Check sheet for the modelled part. Datum: model origin and axes. Units: mm. A direction names the side the tool comes from. Give positions to 0.01 mm unless a question says otherwise; leave off trailing zeros. Write each loop counter-clockwise with the first axis right and the second up, starting at its lowest first coordinate (ties: lowest second). Pieces come first, ordered by that corner, then holes. Notation, with made-up numbers: M -23.5,-6 L -1.5,-6 A21 ccw -1.5,5 Z; hole C 37.5,56 d8. An arc over 180 degrees is marked long. One line per item, written item: value. Start each with the question number.
from build123d import *

# Parameters (mm, degrees)
SKETCH1_R           = 11
BOSS_EXTRUDE1_DEPTH = 36.1
SKETCH3_R           = 2.15
CUT_EXTRUDE1_DEPTH  = 17


with BuildPart() as part:
    # Sketch1 → Boss-Extrude1 (new body)
    with BuildSketch(Plane.XY):
        Polygon((-15, 15), (15, 15), (25, 15), (25, 5), (25, -15), (-25, -15), (-25, 5), (-25, 15), align=None)
        Circle(SKETCH1_R, mode=Mode.SUBTRACT)
    extrude(amount=BOSS_EXTRUDE1_DEPTH)

    # Sketch3 → Cut-Extrude1 (cut)
    with BuildSketch(Plane.XZ.offset(15)):
        with Locations((-17.5, 30.05)):
            Circle(SKETCH3_R)
        with Locations((17.5, 30.05)):
            Circle(SKETCH3_R)
        with Locations((17.5, 6.05)):
            Circle(SKETCH3_R)
        with Locations((-17.5, 6.05)):
            Circle(SKETCH3_R)
    extrude(amount=-CUT_EXTRUDE1_DEPTH, mode=Mode.SUBTRACT)


solid = part.part
1) Gauge pin test, flat end, axial feed: pin 1 (1.3 mm diameter, centred on x = -18.5, z = 30.5, fed in from -Y). Record the tip position at first contact, or that the pin passes through.
2) Cross-section at D-D (y = 5.5). Record the boundary of the cut face in (x, z), plus the area to 3 significant figures.
3) Cross-section at A-A (x = 0). Record the boundary of the cut face in (y, z).
4) Draft check along Y on faces 1 (the flat face through (17, 2, 6)), 2 (the cylindrical face through (-2.38, -10.74, 17.8)), 3 (the flat face through (25, 0, 18)). Enter one of: released by +Y, released by -Y, zero draft, split by the parting line, or undercut.
5) Cross-section at C-C (z = 6.05). Record the boundary of the cut face in (x, y), plus the area to 3 significant figures.
6) Tool access check on faces 4 (the cylindrical face through (17.22, -6.62, 32.18)), 5 (the flat face through (11.5, 0.2, 36.1)). Record the directions out of +Z, -Z, +X, -X, +Y, -Y that give a thin tool (end or side, any length) a straight path to the whole face; none if there is none.
7) Material ranges on L1, parallel to Z at x = -17.5, y = -9.25; L2, parallel to Y at x = 0, z = 20.5; L3, parallel to Z at x = -18, y = -12, recorded low to high. Write a range as from..to.
8) Cross-section at B-B (y = -10). Record the boundary of the cut face in (x, z), plus the area to 3 significant figures.
Data:
1. pin 1: stops at y = 2
2. outline: M -25,0 L -9.53,0 L -9.53,36.1 L -25,36.1 Z; M 9.53,0 L 25,0 L 25,36.1 L 9.53,36.1 Z
2. area: 1,120 mm2
3. outline: M -15,0 L -11,0 L -11,36.1 L -15,36.1 Z; M 11,0 L 15,0 L 15,36.1 L 11,36.1 Z
4. face 1: released by -Y
4. face 2: undercut
4. face 3: zero draft
5. outline: M -25,-15 L -19.65,-15 L -19.65,2 L -15.35,2 L -15.35,-15 L 15.35,-15 L 15.35,2 L 19.65,2 L 19.65,-15 L 25,-15 L 25,15 L -25,15 Z; hole C 0,0 d22
5. area: 974 mm2
6. face 4: -Y
6. face 5: +Z, +X, -X, +Y, -Y
7. L1: z = 0..3.9, 8.2..27.9, 32.2..36.1
7. L2: y = -15..-11, 11..15
7. L3: z = 0..3.96, 8.14..27.96, 32.14..36.1
8. outline: M -25,0 L -4.58,0 L -4.58,36.1 L -25,36.1 Z; M 4.58,0 L 25,0 L 25,36.1 L 4.58,36.1 Z; hole C -17.5,6.05 d4.3; hole C -17.5,30.05 d4.3; hole C 17.5,6.05 d4.3; hole C 17.5,30.05 d4.3
8. area: 1,420 mm2
